from build123d import *

# Parameters (mm, degrees)
F0_W     = 609.6
F0_H     = 609.6
F1_DEPTH = 6.35
F3_DEPTH = 304.8
F4_R     = 12.7
F5_DEPTH = 317.501


with BuildPart() as f1:
    # F0 (on Top) → F1 (new body, symmetric)
    with BuildSketch(Plane.XY):
        with Locations((304.8, 304.8)):
            Rectangle(F0_W, F0_H)
    extrude(amount=F1_DEPTH, both=True)

    # F2 (on face) → F3 (join)
    with BuildSketch(Plane(origin=(0, 0, -6.35), x_dir=(1, 0, 0), z_dir=(0, 0, -1))):
        Polygon((19.05, -19.05), (0, -19.05), (0, -31.75), (19.05, -31.75), (19.05, -50.8), (31.75, -50.8), (31.75, -31.75), (50.8, -31.75), (50.8, -19.05), (31.75, -19.05), (31.75, 0), (19.05, 0), align=None)
        Polygon((590.55, -50.8), (590.55, -31.75), (609.6, -31.75), (609.6, -19.05), (590.55, -19.05), (590.55, 0), (577.85, 0), (577.85, -19.05), (558.8, -19.05), (558.8, -31.75), (577.85, -31.75), (577.85, -50.8), align=None)
        Polygon((19.05, -590.55), (19.05, -609.6), (31.75, -609.6), (31.75, -590.55), (50.8, -590.55), (50.8, -577.85), (31.75, -577.85), (31.75, -558.8), (19.05, -558.8), (19.05, -577.85), (0, -577.85), (0, -590.55), align=None)
        Polygon((577.85, -609.6), (590.55, -609.6), (590.55, -590.55), (609.6, -590.55), (609.6, -577.85), (590.55, -577.85), (590.55, -558.8), (577.85, -558.8), (577.85, -577.85), (558.8, -577.85), (558.8, -590.55), (577.85, -590.55), align=None)
    extrude(amount=F3_DEPTH)

    # F4 (on face) → F5 (cut, through all)
    with BuildSketch(Plane.XY.offset(6.35)):
        with Locations((304.8, 304.8)):
            Circle(F4_R)
    extrude(amount=-F5_DEPTH, mode=Mode.SUBTRACT)


solid = f1.part
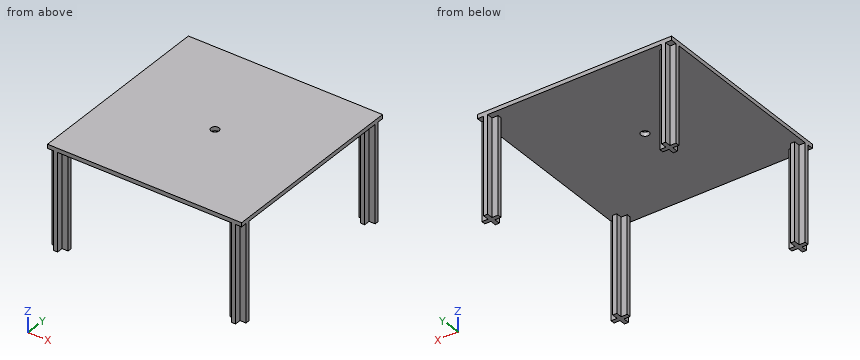
Input: part model. Units: mm. Frame: model coordinates. Coordinates: 2 decimals unless noted, no trailing zeros. Loops run counter-clockwise (first coordinate to the right, second up) from the corner with the lowest first, then second, coordinate; pieces in that order, holes last.
(1) Section A-A on y = 304.8. Return the cut outline in (x, z), then the cut area to 3 significant figures.
(2) Section C-C on z = -210. Count the separate pieces of the cut face and the enclosed holes in it, then the cut area to 3 significant figures.
(3) First-contact query: pin 1 Ø5.5 at (x, z) = (37, -133) entering from +Y; pin 2 Ø5.5 at (x, z) = (7, -122) entering from -Y; pin 3 Ø4 at (x, z) = (583.5, -231) entering from -Y; pin 4 Ø15 at (x, y) = (602.5, 6.5) entering from -Z. Flat tips, straight axial feed; report the tip coordinate or a pass-through.
(4) Section D-D on x = 188.5. Return the cut outline in (y, z), then the cut area to 3 significant figures.
(5) Material intervals for probe 1 along Y at (x, z) = (304.8, 2.5); probe 2 along Y at (x, z) = (30, -204.5); probe 3 along X at (y, z) = (560.5, -202), sorted ascending.
Data:
1. outline: (0, -6.35) - (292.1, -6.35) - (292.1, 6.35) - (0, 6.35) - close; (317.5, -6.35) - (609.6, -6.35) - (609.6, 6.35) - (317.5, 6.35) - close
1. area: 7,420 mm2
2. separate pieces: 4
2. enclosed holes: 0
2. area: 4,520 mm2
3. pin 1: stops at y = 590.55
3. pin 2: stops at y = 19.05
3. pin 3: stops at y = 0
3. pin 4: stops at z = -6.35
4. outline: (0, -6.35) - (609.6, -6.35) - (609.6, 6.35) - (0, 6.35) - close
4. area: 7,740 mm2
5. probe 1: y = 0 to 292.1, 317.5 to 609.6
5. probe 2: y = 0 to 50.8, 558.8 to 609.6
5. probe 3: x = 19.05 to 31.75, 577.85 to 590.55
